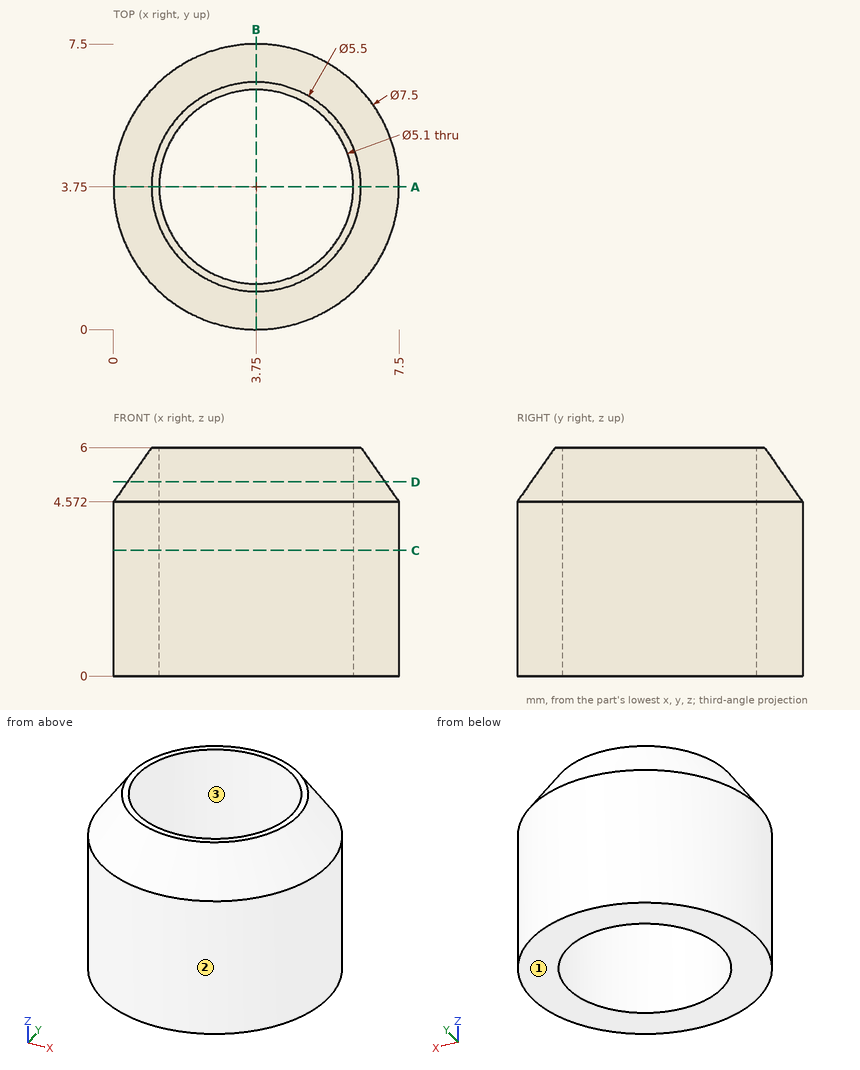
Job drawing, mm, ordinate dimensions from the low corner. One solid piece. Coordinates: 2 decimals unless noted, no trailing zeros. Order: outer loops, then holes, each group sorted by start corner. A loop starts at its lowest first (then second) coordinate and runs counter-clockwise, first axis right, second up. Notation, with made-up numbers: (43, 78.5) -> (55, 78.5) arc R16 ccw to (55, 92.5) -> close; hole circle Ø4 at (-39, 5). An arc over 180 degrees is marked (long way). Return JSON: item names as keys, results as strings. Group by question number.
Item 1: Saw through at D-D on z = 5.1. Write the cut outline in (x, y).
Item 2: Pull direction Y, two halves, no side cores. Call the marked faces 1, 2 and 3: pulls with the +Y half, pulls with the -Y half, needs draft (parallel to the pull), parting line crosses it, or undercut.
Item 3: Wall check: line 1 along Y through (x, z) = (3.75, 2.35); line 2 along Y through (x, z) = (5, 2.05) (1 decimal); line 3 along X through (y, z) = (6.5, 1.7). Give the ranges that are in metal, low to high. Write a range as [from, to].
Item 4: Flat gauge pins, fed straight in: P1, Ø4.5, axis at x = 3.75, y = 3.75, coming from the -Z side; P2, Ø1, axis at x = 1.5, z = 3.5, coming from the -Y side. Where does each tip first touch, or does it go through?
Item 5: Saw through at C-C on z = 3.3. Write the cut outline in (x, y).
Item 6: Saw through at A-A on y = 3.75. Write the cut outline in (x, z), then the cut area to 3 significant figures.
Values found:
{
 "1": {"outline": "circle Ø6.76 at (3.75, 3.75); hole circle Ø5.1 at (3.75, 3.75)"},
 "2": {"face 1": "needs draft", "face 2": "parting line crosses it", "face 3": "undercut"},
 "3": {"line 1": "y = [0, 1.2], [6.3, 7.5]", "line 2": "y = [0.2, 1.5], [6, 7.3]", "line 3": "x = [1.2, 6.3]"},
 "4": {"P1": "passes through", "P2": "stops at y = 0.43"},
 "5": {"outline": "circle Ø7.5 at (3.75, 3.75); hole circle Ø5.1 at (3.75, 3.75)"},
 "6": {"outline": "(0, 0) -> (1.2, 0) -> (1.2, 6) -> (1, 6) -> (0, 4.57) -> close; (6.3, 0) -> (7.5, 0) -> (7.5, 4.57) -> (6.5, 6) -> (6.3, 6) -> close", "area": "13.0 mm2"}
}
